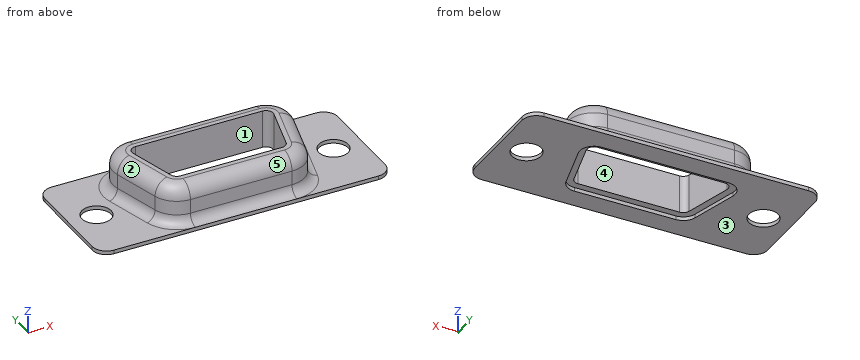
from build123d import *

# Parameters (mm, degrees)
SKETCH1_R           = 1.55
BOSS_EXTRUDE1_DEPTH = 0.4
BOSS_EXTRUDE2_DEPTH = 4
FILLET1_R           = 1
FILLET2_R           = 1.5


with BuildPart() as part:
    # Sketch1 → Boss-Extrude1 (new body)
    with BuildSketch(Plane.XY):
        with BuildLine():
            Line((13.95, 6.25), (-13.95, 6.25))
            ThreePointArc((-13.95, 6.25), (-15.010660172, 5.810660172), (-15.45, 4.75))
            Line((-15.45, 4.75), (-15.45, -4.75))
            ThreePointArc((-15.45, -4.75), (-15.010660172, -5.810660172), (-13.95, -6.25))
            Line((-13.95, -6.25), (13.95, -6.25))
            ThreePointArc((13.95, -6.25), (15.010660172, -5.810660172), (15.45, -4.75))
            Line((15.45, -4.75), (15.45, 4.75))
            ThreePointArc((15.45, 4.75), (15.010660172, 5.810660172), (13.95, 6.25))
        make_face()
        with Locations((-12.5, 0)):
            Circle(SKETCH1_R, mode=Mode.SUBTRACT)
        with BuildLine():
            Line((-6.806228507, -2.888228568), (-8.145974469, 2.111771432))
            ThreePointArc((-8.145974469, 2.111771432), (-7.88711574, 3.413142144), (-6.697085729, 4))
            Line((-6.697085729, 4), (6.697085729, 4))
            ThreePointArc((6.697085729, 4), (7.88711574, 3.413142144), (8.145974469, 2.111771432))
            Line((8.145974469, 2.111771432), (6.806228507, -2.888228568))
            ThreePointArc((6.806228507, -2.888228568), (6.270481911, -3.69003001), (5.357339767, -4))
            Line((5.357339767, -4), (-5.357339767, -4))
            ThreePointArc((-5.357339767, -4), (-6.270481911, -3.69003001), (-6.806228507, -2.888228568))
        make_face(mode=Mode.SUBTRACT)
        with Locations((12.5, 0)):
            Circle(SKETCH1_R, mode=Mode.SUBTRACT)
    extrude(amount=BOSS_EXTRUDE1_DEPTH)

    # Sketch2 → Boss-Extrude2 (add)
    with BuildSketch(Plane.XY.offset(0.4)):
        with BuildLine():
            Line((-9.353381752, 1.788247626), (-8.01363579, -3.211752374))
            ThreePointArc((-8.01363579, -3.211752374), (-7.031433697, -4.681721686), (-5.357339767, -5.25))
            Line((-5.357339767, -5.25), (5.357339767, -5.25))
            ThreePointArc((5.357339767, -5.25), (7.031433697, -4.681721686), (8.01363579, -3.211752374))
            Line((8.01363579, -3.211752374), (9.353381752, 1.788247626))
            ThreePointArc((9.353381752, 1.788247626), (8.878807415, 4.17409393), (6.697085729, 5.25))
            Line((6.697085729, 5.25), (-6.697085729, 5.25))
            ThreePointArc((-6.697085729, 5.25), (-8.878807415, 4.17409393), (-9.353381752, 1.788247626))
        make_face()
        with BuildLine():
            Line((-5.357339767, -3.25), (5.357339767, -3.25))
            ThreePointArc((5.357339767, -3.25), (5.813910839, -3.095015005), (6.081784137, -2.694114284))
            Line((6.081784137, -2.694114284), (7.421530099, 2.305885716))
            ThreePointArc((7.421530099, 2.305885716), (7.292100735, 2.956571072), (6.697085729, 3.25))
            Line((6.697085729, 3.25), (-6.697085729, 3.25))
            ThreePointArc((-6.697085729, 3.25), (-7.292100735, 2.956571072), (-7.421530099, 2.305885716))
            Line((-7.421530099, 2.305885716), (-6.081784137, -2.694114284))
            ThreePointArc((-6.081784137, -2.694114284), (-5.813910839, -3.095015005), (-5.357339767, -3.25))
        make_face(mode=Mode.SUBTRACT)
    extrude(amount=BOSS_EXTRUDE2_DEPTH)

    # Fillet1
    fillet1_edges = [part.edges().sort_by_distance(p)[0] for p in [
        (-8.878807415, 4.17409393, 0.4),
        (-8.683508771, -0.711752374, 0.4),
        (-7.031433697, -4.681721686, 0.4),
        (0, -5.25, 0.4),
        (7.031433697, -4.681721686, 0.4),
        (8.683508771, -0.711752374, 0.4),
        (8.878807415, 4.17409393, 0.4),
        (0, 5.25, 0.4),
    ]]
    fillet(fillet1_edges, radius=FILLET1_R - 0.0001)  # a hair under: the kernel refuses the full size

    # Fillet2
    fillet2_edges = [part.edges().sort_by_distance(p)[0] for p in [
        (-8.878807415, 4.17409393, 4.4),
        (-8.683508771, -0.711752374, 4.4),
        (-7.031433697, -4.681721686, 4.4),
        (0, -5.25, 4.4),
        (7.031433697, -4.681721686, 4.4),
        (8.683508771, -0.711752374, 4.4),
        (8.878807415, 4.17409393, 4.4),
        (0, 5.25, 4.4),
    ]]
    fillet(fillet2_edges, radius=FILLET2_R)


solid = part.part
For this review, take the finished solid that the model builds, in its own axes (mm). Face numbers are marked on the shaded views. A direction names the side the tool comes from. Give positions to 0.01 mm unless a question says otherwise; leave off trailing zeros. Order: outer loops, then holes, each group sorted by start corner. A loop starts at its lowest first (then second) coordinate and runs counter-clockwise, first axis right, second up. Notation, with made-up numbers: (41.5, -25) -> (81.5, -25) arc R20 ccw to (81.5, 13) -> close; hole circle Ø11 at (-13, 25). An arc over 180 degrees is marked (long way). Write item = value, one per line.
1) Insertion check: pin 1 (1.2 mm diameter, centred on x = 1.5, z = 2, fed in from -Y); pin 2 (0.8 mm diameter, centred on x = -3.5, z = 2, fed in from +Y); pin 3 (4 mm diameter, centred on x = 11, y = 3, fed in from +Z). Each pin has a flat end and moves straight along its axis. Give the tip position at first contact, or say it passes through.
Findings:
pin_1 = -5.25
pin_2 = 5.25
pin_3 = 3.94
2) We need section B-B, the plane z = 2.2. Give the boundary of the cut face in (x, y).
Findings:
outline = (-9.35, 1.79) -> (-8.01, -3.21) arc R2.75 ccw to (-5.36, -5.25) -> (5.36, -5.25) arc R2.75 ccw to (8.01, -3.21) -> (9.35, 1.79) arc R2.75 ccw to (6.7, 5.25) -> (-6.7, 5.25) arc R2.75 ccw to start; hole (-7.42, 2.31) -> (-6.08, -2.69) arc R0.75 ccw to (-5.36, -3.25) -> (5.36, -3.25) arc R0.75 ccw to (6.08, -2.69) -> (7.42, 2.31) arc R0.75 ccw to (6.7, 3.25) -> (-6.7, 3.25) arc R0.75 ccw to start
3) We need section A-A, the plane x = 12.5. Give the boundary of the cut face in (y, z).
Findings:
outline = (-6.25, 0) -> (-1.55, 0) -> (-1.55, 0.4) -> (-6.25, 0.4) -> close; (1.55, 0) -> (6.25, 0) -> (6.25, 0.4) -> (1.55, 0.4) -> close
4) We need section C-C, the plane y = 0. Count the separate pieces of the cut face and the enclosed holes in it, and give its area (3 significant figures).
Findings:
separate_pieces = 4
enclosed_holes = 0
area = 19.8 mm^2
5) Draft analysis for pull direction Y (two halves, no side actions). For the marked faces 1, 2 and 3, state which applies: pulls with the +Y half, pulls with the -Y half, needs draft (parallel to the pull), parting line crosses it, or undercut.
Findings:
face_1 = undercut
face_2 = pulls with the -Y half
face_3 = needs draft
6) We need section D-D, the plane z = 1. Give the boundary of the cut face in (x, y), and give its area (3 significant figures).
Findings:
outline = (-9.43, 1.77) -> (-8.09, -3.23) arc R2.83 ccw to (-5.36, -5.33) -> (5.36, -5.33) arc R2.83 ccw to (8.09, -3.23) -> (9.43, 1.77) arc R2.83 ccw to (6.7, 5.33) -> (-6.7, 5.33) arc R2.83 ccw to start; hole (-7.42, 2.31) -> (-6.08, -2.69) arc R0.75 ccw to (-5.36, -3.25) -> (5.36, -3.25) arc R0.75 ccw to (6.08, -2.69) -> (7.42, 2.31) arc R0.75 ccw to (6.7, 3.25) -> (-6.7, 3.25) arc R0.75 ccw to start
area = 95.3 mm^2
7) For the marked faces 4 and 5, list the 3-axis set-ups (+Z, -Z, +X, -X, +Y, -Y) from which the entire face can be reached by the end or side of a thin tool; tool diameter is ignored.
Findings:
face_4 = +Z, -Z
face_5 = +Z, +X, -X, -Y
8) To check wall thickness, follow L1, parallel to Y at x = -12.5, z = 0.1; L2, parallel to Y at x = -0.5, z = 2.1; L3, parallel to Z at x = 13, y = 4.5. State the ranges of each line that lie inside material, in increasing order. Write a range as from..to.
Findings:
L1 = -6.25..-1.55, 1.55..6.25
L2 = -5.25..-3.25, 3.25..5.25
L3 = 0..0.4
